Part print with two shaded views. Sizes in mm from the minimum x, y, z corner. A direction names the side the tool comes from. Coordinates: 2 decimals unless noted, no trailing zeros. Write each loop counter-clockwise with the first axis right and the second up, starting at its lowest first coordinate (ties: lowest second). Pieces come first, ordered by that corner, then holes. Notation, with made-up numbers: (17.5, 28.5) - (27.5, 28.5) arc R14 cw to (27.5, 38.5) - close; hole circle Ø10 at (-2.75, 69). An arc over 180 degrees is marked (long way). Answer in a Markdown table with one row per item. Add a question column.
Q1. 3-axis set-ups, long thin cutter, end or side, ignore diameter. For the marked faces 1 and 2: which of +Z, -Z, +X, -X, +Y, -Y reach the whole face in a straight line?
Q2. Band-saw the part on A-A (x = 5.85). List the corners of the cut face in (y, z), and give its area (3 significant figures).
Q3. Pin check, flat tips, straight feed: pin 1 (2 mm diameter, centred on y = 8, z = 30.5, fed in from -X); pin 2 (6 mm diameter, centred on y = 2.5, z = 25.5, fed in from +X); pin 3 (4 mm diameter, centred on x = 5.5, z = 16, fed in from -Y). Stop position of each tip, or through.
Q4. Drill centre lines: line 1 along Z through (x, y) = (8.25, 8.75); line 2 along Y through (x, z) = (6, 17); line 3 along Z through (x, y) = (4.5, 8.75). Where is each one in solid material? Low to high. Write a range as from..to.
Q5. Band-saw the part on C-C (z = 14). List the corners of the cut face in (x, y).
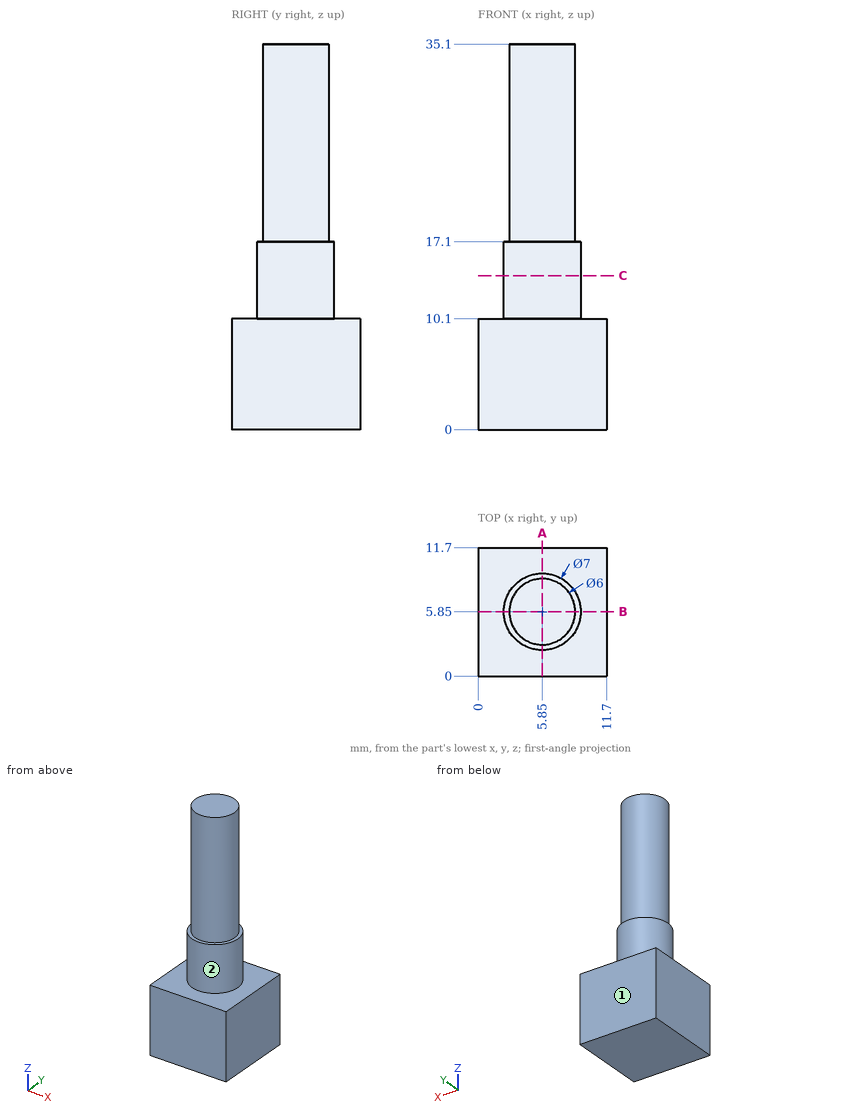
Checked values:
| question | item | result |
|---|---|---|
| 1 | face 1 | +Z, -Z, +X, -X, +Y |
| 1 | face 2 | +Z |
| 2 | outline | (0, 0) - (11.7, 0) - (11.7, 10.1) - (9.35, 10.1) - (9.35, 17.1) - (8.85, 17.1) - (8.85, 35.1) - (2.85, 35.1) - (2.85, 17.1) - (2.35, 17.1) - (2.35, 10.1) - (0, 10.1) - close |
| 2 | area | 275 mm² |
| 3 | pin 1 | stops at x = 3.08 |
| 3 | pin 2 | stops at x = 8.83 |
| 3 | pin 3 | stops at y = 2.35 |
| 4 | line 1 | z = 0..10.1 |
| 4 | line 2 | y = 2.35..9.35 |
| 4 | line 3 | z = 0..17.1 |
| 5 | outline | circle Ø7 at (5.85, 5.85) |
